```python
from build123d import *

# Parameters (mm, degrees)
BOSS_EXTRUDE1_DEPTH  = 5
SKETCH2_W            = 55.5
SKETCH2_H            = 33.15
CUT_EXTRUDE1_DEPTH   = 10
SKETCH3_W            = 59.5
SKETCH3_H            = 37.15
CUT_EXTRUDE2_DEPTH   = 2.5
SKETCH4_R            = 13.5
CUT_EXTRUDE3_DEPTH   = 2.5
SKETCH8_W            = 89
SKETCH8_H            = 36.5
CUT_EXTRUDE4_DEPTH   = 2.5
BOSS_EXTRUDE4_DEPTH  = 105
SKETCH10_OUTSIDE_W   = 200.486
SKETCH10_OUTSIDE_H   = 145.486
CUT_EXTRUDE5_DEPTH   = 105
SKETCH5_R            = 1.35
SKETCH5_R_2          = 0.95
SKETCH5_R_3          = 1.2
CUT_EXTRUDE6_DEPTH   = 3
SKETCH11_OUTSIDE_W   = 200.486
SKETCH11_OUTSIDE_H   = 145.486
SKETCH11_OUTSIDE_W_2 = 65.5
SKETCH11_OUTSIDE_H_2 = 43.15
CUT_EXTRUDE7_DEPTH   = 10


with BuildPart() as part:
    # Sketch1 → Boss-Extrude1 (new body)
    with BuildSketch(Plane(origin=(0, 0, 0), x_dir=(1, 0, 0), z_dir=(0, 1, 0))):
        with BuildLine():
            Line((40, -52.5), (-40, -52.5))
            ThreePointArc((-40, -52.5), (-68.284271247, -40.784271247), (-80, -12.5))
            Line((-80, -12.5), (-80, 12.5))
            ThreePointArc((-80, 12.5), (-68.284271247, 40.784271247), (-40, 52.5))
            Line((-40, 52.5), (40, 52.5))
            ThreePointArc((40, 52.5), (68.284271247, 40.784271247), (80, 12.5))
            Line((80, 12.5), (80, -12.5))
            ThreePointArc((80, -12.5), (68.284271247, -40.784271247), (40, -52.5))
        make_face()
    extrude(amount=BOSS_EXTRUDE1_DEPTH)

    # Sketch2 → Cut-Extrude1 (cut)
    with BuildSketch(Plane(origin=(0, 0, 0), x_dir=(-1, 0, 0), z_dir=(0, -1, 0))):
        with Locations((-6.459334532, -28.560438218)):
            Rectangle(SKETCH2_W, SKETCH2_H)
    extrude(amount=-CUT_EXTRUDE1_DEPTH, mode=Mode.SUBTRACT)

    # Sketch3 → Cut-Extrude2 (cut)
    with BuildSketch(Plane(origin=(0, 5, 0), x_dir=(1, 0, 0), z_dir=(0, 1, 0))):
        with Locations((6.459334532, -28.560438218)):
            Rectangle(SKETCH3_W, SKETCH3_H)
    extrude(amount=-CUT_EXTRUDE2_DEPTH, mode=Mode.SUBTRACT)

    # Sketch4 → Cut-Extrude3 (cut)
    with BuildSketch(Plane(origin=(0, 5, 0), x_dir=(1, 0, 0), z_dir=(0, 1, 0))):
        with Locations(Location((56.229894871, -16.5, 0), (0, 0, 270))):
            Circle(SKETCH4_R)
        with Locations(Location((-56.229894871, -16.5, 0), (0, 0, 90))):
            Circle(SKETCH4_R)
    extrude(amount=-CUT_EXTRUDE3_DEPTH, mode=Mode.SUBTRACT)

    # Sketch8 → Cut-Extrude4 (cut)
    with BuildSketch(Plane(origin=(0, 5, 0), x_dir=(1, 0, 0), z_dir=(0, 1, 0))):
        with Locations((0.079334532, 25.25)):
            Rectangle(SKETCH8_W, SKETCH8_H)
    extrude(amount=-CUT_EXTRUDE4_DEPTH, mode=Mode.SUBTRACT)

    # Sketch9 → Boss-Extrude4 (add)
    with BuildSketch(Plane.XY.offset(52.5)):
        with BuildLine():
            Line((-80, 0), (-40, 0))
            add(Edge.make_bspline(
                [(-80, 0), (-79.948023713, -3.673692429), (-77.584130198, -11.396455763), (-57.110208015, -20.509844228), (-48.902789398, -1.350898332), (-40, 0)],
                knots=[0, 0, 0, 0, 0.184459574, 0.474643138, 1, 1, 1, 1], degree=3))
        make_face()
        with BuildLine():
            Line((40, 0), (80, 0))
            add(Edge.make_bspline(
                [(80, 0), (79.948023713, -3.673692429), (77.584130198, -11.396455763), (57.110208015, -20.509844228), (48.902789398, -1.350898332), (40, 0)],
                knots=[0, 0, 0, 0, 0.184459574, 0.474643138, 1, 1, 1, 1], degree=3))
        make_face()
    extrude(amount=-BOSS_EXTRUDE4_DEPTH)

    # Sketch10 outside → Cut-Extrude5 (cut)
    with BuildSketch(Plane(origin=(0, 5, 0), x_dir=(1, 0, 0), z_dir=(0, 1, 0))):
        Rectangle(SKETCH10_OUTSIDE_W, SKETCH10_OUTSIDE_H)
        with BuildLine():
            Line((-80, 12.5), (-80, -12.5))
            ThreePointArc((-80, -12.5), (-68.284271247, -40.784271247), (-40, -52.5))
            Line((-40, -52.5), (40, -52.5))
            ThreePointArc((40, -52.5), (68.284271247, -40.784271247), (80, -12.5))
            Line((80, -12.5), (80, 12.5))
            ThreePointArc((80, 12.5), (68.284271247, 40.784271247), (40, 52.5))
            Line((40, 52.5), (-40, 52.5))
            ThreePointArc((-40, 52.5), (-68.284271247, 40.784271247), (-80, 12.5))
        make_face(mode=Mode.SUBTRACT)
    extrude(amount=-CUT_EXTRUDE5_DEPTH, mode=Mode.SUBTRACT)

    # Sketch5 → Cut-Extrude6 (cut)
    with BuildSketch(Plane(origin=(0, 5, 0), x_dir=(1, 0, 0), z_dir=(0, 1, 0))):
        with Locations(Location((66.054894871, -29.425, 0), (0, 0, 270))):
            Circle(SKETCH5_R)
        with Locations(Location((46.404894871, -29.425, 0), (0, 0, 270))):
            Circle(SKETCH5_R)
        with Locations(Location((66.054894871, -3.575, 0), (0, 0, 270))):
            Circle(SKETCH5_R)
        with Locations(Location((46.404894871, -3.575, 0), (0, 0, 270))):
            Circle(SKETCH5_R)
        with Locations(Location((-46.404894871, -29.425, 0), (0, 0, 90))):
            Circle(SKETCH5_R)
        with Locations(Location((-66.054894871, -29.425, 0), (0, 0, 90))):
            Circle(SKETCH5_R)
        with Locations(Location((-66.054894871, -3.575, 0), (0, 0, 90))):
            Circle(SKETCH5_R)
        with Locations(Location((-46.404894871, -3.575, 0), (0, 0, 90))):
            Circle(SKETCH5_R)
        with Locations(Location((46.579334532, 44.5, 0), (0, 0, 270))):
            Circle(SKETCH5_R_2)
        with Locations(Location((46.579334532, 5, 0), (0, 0, 270))):
            Circle(SKETCH5_R_2)
        with Locations(Location((-46.420665468, 5, 0), (0, 0, 270))):
            Circle(SKETCH5_R_2)
        with Locations(Location((-46.420665468, 44.5, 0), (0, 0, 270))):
            Circle(SKETCH5_R_2)
        with Locations(Location((-29.520665468, 0.75, 0), (0, 0, 270))):
            Circle(SKETCH5_R_3)
        with Locations(Location((-29.520665468, -44.95, 0), (0, 0, 270))):
            Circle(SKETCH5_R_3)
        with Locations(Location((36.179334532, 0.75, 0), (0, 0, 270))):
            Circle(SKETCH5_R_3)
    extrude(amount=-CUT_EXTRUDE6_DEPTH, mode=Mode.SUBTRACT)

    # Sketch11 outside → Cut-Extrude7 (cut)
    with BuildSketch(Plane(origin=(0, 5, 0), x_dir=(1, 0, 0), z_dir=(0, 1, 0))):
        Rectangle(SKETCH11_OUTSIDE_W, SKETCH11_OUTSIDE_H)
        with Locations((6.459334532, -28.560438218)):
            Rectangle(SKETCH11_OUTSIDE_W_2, SKETCH11_OUTSIDE_H_2, mode=Mode.SUBTRACT)
    extrude(amount=-CUT_EXTRUDE7_DEPTH, mode=Mode.SUBTRACT)


with BuildPart() as cut_extrude7_kept_piece:
    # of the separate pieces the step leaves, the one the design keeps (cut_extrude7_pieces_kept)
    add(part.part.solids().sort_by_distance((39.209334532, 0, 6.985438218))[0])


solid = cut_extrude7_kept_piece.part
```
Part model, mm, in its own coordinate system. A direction names the side the tool comes from. Round coordinates to 2 decimals unless told otherwise and drop trailing zeros. Loops run counter-clockwise (first coordinate to the right, second up) from the corner with the lowest first, then second, coordinate; pieces in that order, holes last. Notation, with made-up numbers: (-22, 58) -> (4, 58) arc R11 ccw to (4, 73) -> close; hole circle Ø11 at (-12.5, 23). An arc over 180 degrees is marked (long way). Use one line per item in the form item = value. Start each with the question number.
Item 1: Tool access for faces 4 (the flat face through (-23.291, 4, 29)), 5 (the flat face through (7, 0, 47)), 6 (the flat face through (-21.291, 1, 29)): list every direction of +Z, -Z, +X, -X, +Y, -Y with a clear straight run to the whole face (end or side of a thin tool).
Item 2: Band-saw the part on A-A (y = 3.9). List the corners of the cut face in (x, z).
Item 3: Band-saw the part on D-D (y = 1). List the corners of the cut face in (x, z).
Item 4: Band-saw the part on B-B (x = -3). List the corners of the cut face in (y, z), plus the area to 3 significant figures.
Item 5: Band-saw the part on C-C (z = 44.5). List the corners of the cut face in (x, y), plus the area to 3 significant figures.
Item 6: Two-plate mould, pull along Z, no slides. Class faces 1 (the flat face through (6, 3, 6.985)), 2 (the flat face through (7, 1, 45.135)), 3 (the flat face through (-26.291, 3, 29)): released by +Z, released by -Z, zero draft, split by the parting line, or undercut.
Item 7: Drill centre lines: line 1 along Z through (x, y) = (12.5, 2.6); line 2 along Z through (x, y) = (12, 1.15); line 3 along X through (y, z) = (4.15, 23.5). Where is each one in solid material? Low to high.
Data:
q1.face_4 = +Y
q1.face_5 = +Z, -Z, +X, -X, -Y
q1.face_6 = +Y, -Y
q2.outline = (-26.29, 6.99) -> (39.21, 6.99) -> (39.21, 50.14) -> (-26.29, 50.14) -> close; hole (-23.29, 9.99) -> (36.21, 9.99) -> (36.21, 47.14) -> (-23.29, 47.14) -> close
q3.outline = (-26.29, 6.99) -> (39.21, 6.99) -> (39.21, 50.14) -> (-26.29, 50.14) -> close; hole (-21.29, 11.99) -> (34.21, 11.99) -> (34.21, 45.14) -> (-21.29, 45.14) -> close
q4.outline = (0, 6.99) -> (5, 6.99) -> (5, 9.99) -> (2.5, 9.99) -> (2.5, 11.99) -> (0, 11.99) -> close; (0, 45.14) -> (2.5, 45.14) -> (2.5, 47.14) -> (5, 47.14) -> (5, 50.14) -> (0, 50.14) -> close
q4.area = 40.0 mm^2
q5.outline = (-26.29, 0) -> (-21.29, 0) -> (-21.29, 2.5) -> (-23.29, 2.5) -> (-23.29, 5) -> (-26.29, 5) -> close; (34.21, 0) -> (39.21, 0) -> (39.21, 5) -> (36.21, 5) -> (36.21, 2.5) -> (34.21, 2.5) -> close
q5.area = 40.0 mm^2
q6.face_1 = released by -Z
q6.face_2 = undercut
q6.face_3 = zero draft
q7.line_1 = 6.99 to 9.99, 47.14 to 50.14
q7.line_2 = 6.99 to 11.99, 45.14 to 50.14
q7.line_3 = -26.29 to -23.29, 36.21 to 39.21
